Check sheet for the modelled part. Datum: model origin and axes. Units: mm. A direction names the side the tool comes from. Give positions to 0.01 mm unless a question says otherwise; leave off trailing zeros. Loops run counter-clockwise (first coordinate to the right, second up) from the corner with the lowest first, then second, coordinate; pieces in that order, holes last. Notation, with made-up numbers: (0.5, 23.5) -> (52.5, 23.5) arc R28 ccw to (52.5, 49.5) -> close; hole circle Ø5 at (-33, 1). An arc over 180 degrees is marked (long way). Write each question's results on one line, items separated by ' | '. Start each with the question number.
1. Material ranges on L1, parallel to Y at x = 83.5, z = 10; L2, parallel to X at y = 9.5, z = -4; L3, parallel to Z at x = 19, y = 0, recorded low to high. Write a range as from..to.
2. Tool access check on faces 4 (the face through (89, -20, 0)), 5 (the face through (60, -5, 5)). Record the directions out of +Z, -Z, +X, -X, +Y, -Y that give a thin tool (end or side, any length) a straight path to the whole face; none if there is none.
3. Cross-section at A-A on z = 11.5. Record the boundary of the cut face in (x, y), and give its area (3 significant figures).
4. Gauge pin test, flat end, axial feed: pin 1 Ø5.5 at (x, y) = (48.5, 7.5) entering from +Z. Record the tip position at first contact, or that the pin passes through.
5. Cross-section at B-B on x = 62.5. Record the boundary of the cut face in (y, z), and give its area (3 significant figures).
6. Mould release check, pull along Y, two halves, no side actions. Record for faces 1 (the face through (7, 4, 5)), 2 (the face through (89, 20, 0)), 3 (the face through (0, 0, 0)): +Y half, -Y half, draft (parallel to the pull), parting line (faces both ways), or undercut.
from build123d import *

# Parameters (mm, degrees)
F0_W     = 40
F0_H     = 30
F1_DEPTH = 180
F3_DEPTH = 20
F4_SIZE  = 1


with BuildPart() as f1:
    # F0 (on Right) → F1 (new body)
    with BuildSketch(Plane.YZ):
        Rectangle(F0_W, F0_H)
    extrude(amount=F1_DEPTH)

    # F2 (on face) → F3 (cut)
    with BuildSketch(Plane.XY.offset(15)):
        with BuildLine():
            Line((10, -5), (112, -5))
            ThreePointArc((112, -5), (114.1213203436, -4.1213203436), (115, -2))
            Line((115, -2), (115, 10))
            ThreePointArc((115, 10), (114.1213203436, 12.1213203436), (112, 13))
            Line((112, 13), (10, 13))
            ThreePointArc((10, 13), (7.8786796564, 12.1213203436), (7, 10))
            Line((7, 10), (7, -2))
            ThreePointArc((7, -2), (7.8786796564, -4.1213203436), (10, -5))
        make_face()
    extrude(amount=-F3_DEPTH, mode=Mode.SUBTRACT)

    # F4
    f4_edges = [f1.edges().sort_by_distance(p)[0] for p in [
        (90, 20, -15),
        (90, 20, 15),
        (0, 20, 0),
        (180, 20, 0),
        (0, 0, 15),
        (0, -20, 0),
        (0, 0, -15),
        (90, -20, 15),
        (180, 0, 15),
        (61, 13, 15),
        (115, 4, 15),
        (180, -20, 0),
        (90, -20, -15),
        (7.87868, 12.12132, 15),
        (114.12132, 12.12132, 15),
        (114.12132, -4.12132, 15),
        (61, -5, 15),
        (7.87868, -4.12132, 15),
        (7, 4, 15),
        (180, 0, -15),
    ]]
    chamfer(f4_edges, length=F4_SIZE)


solid = f1.part
Geometry says:
1) L1: -20..-5, 13..20 | L2: 0..7, 115..180 | L3: -15..-5
2) face 4: +Z, -Z, +X, -X, -Y | face 5: +Z
3) outline: (0, -19) -> (1, -20) -> (179, -20) -> (180, -19) -> (180, 19) -> (179, 20) -> (1, 20) -> (0, 19) -> close; hole (7, -2) arc R3 ccw to (10, -5) -> (112, -5) arc R3 ccw to (115, -2) -> (115, 10) arc R3 ccw to (112, 13) -> (10, 13) arc R3 ccw to (7, 10) -> close | area: 5,260 mm^2
4) pin 1: z = -5
5) outline: (-20, -14) -> (-19, -15) -> (19, -15) -> (20, -14) -> (20, 14) -> (19, 15) -> (14, 15) -> (13, 14) -> (13, -5) -> (-5, -5) -> (-5, 14) -> (-6, 15) -> (-19, 15) -> (-20, 14) -> close | area: 837 mm^2
6) face 1: undercut | face 2: +Y half | face 3: draft
